The listing builds one solid part. Answer for the finished solid, in the listing's coordinates (mm). A direction names the side the tool comes from. Give positions to 0.01 mm unless a question says otherwise; leave off trailing zeros. Loops run counter-clockwise (first coordinate to the right, second up) from the corner with the lowest first, then second, coordinate; pieces in that order, holes last. Notation, with made-up numbers: M -39.5,22.25 L -5.5,22.25 A28 cw -5.5,44.25 Z; hole C 13.25,59 d6. An arc over 180 degrees is marked long. Use one line per item in the form item = value. Start each with the question number.
1. The part is cut by section C-C (y = -4.5). Write down the section's boundary in (x, z), and give its area (3 significant figures).
2. The part is cut by section D-D (z = -25.5). Write down the section's boundary in (x, y), and give its area (3 significant figures).
3. The part is cut by section A-A (x = -39). Write down the section's boundary in (y, z), and give its area (3 significant figures).
4. Each of these flat-tipped pins is pushed along its axis until it touches: pin 1 Ø3 at (y, z) = (-6.5, -50) entering from +X; pin 2 Ø6 at (y, z) = (-6.5, -80.5) entering from +X; pin 3 Ø19.5 at (x, z) = (39, -25.5) entering from +Y; pin 4 Ø6 at (y, z) = (-7, -113.5) entering from -X. Where does it stop, or does it pass through?
5. The part is cut by section B-B (z = -117.5). Write down the section's boundary in (x, y).
6. For faces 1 (the face through (29, -6, -129.5)), 2 (the face through (68.797, -6.084, -1.141)), 3 (the face through (-17, -6, -105.5)), 4 (the face through (50.5, -6, -89)), 5 (the face through (-50.5, -6, -89)), determine the directions among +Z, -Z, +X, -X, +Y, -Y from which every point of the face is accessible in a straight line to the end or side of a thin tool.
7. Straight lines are drawn through the part: line 1 (Z direction, x = -15.5, y = -8.75); line 2 (X direction, y = -1.5, z = -25); line 3 (Z direction, x = 26.5, y = -4.5). For each, find the intervals that lie inside material, in ascending order. Write a range as from..to.
8. The mould has two halves that part along Z. Classify faces 6 (the face through (-11.5, -6, -118)), 7 (the face through (51.703, -6.084, -51.141)), 8 (the face through (0, -6, -84.6)), 9 (the face through (27.216, -5.916, -112.047)): released by +Z, released by -Z, zero draft, split by the parting line, or undercut.
from build123d import *

# Parameters (mm, degrees)
F0_R     = 5.5
F0_R_2   = 7.55
F1_DEPTH = 12
F2_R     = 4


with BuildPart() as f1:
    # F0 (on Front) → F1 (new body)
    with BuildSketch(Plane.XZ):
        Polygon((0, -84.6), (0, 0), (-70, 0), (-70, -50), (-50.5, -50), (-50.5, -129.5), (-11.5, -129.5), (-11.5, -105.5), (-22.5, -105.5), (-22.5, -84.6), align=None)
        with Locations((-26.5, -117.5)):
            Circle(F0_R, mode=Mode.SUBTRACT)
        with Locations((-39, -25.5)):
            Circle(F0_R_2, mode=Mode.SUBTRACT)
    extrude(amount=F1_DEPTH)

    # F2
    f2_edges = [f1.edges().sort_by_distance(p)[0] for p in [
        (-50.5, -6, -129.5),
        (-50.5, -6, -50),
        (-70, -6, -50),
        (-70, -6, 0),
    ]]
    fillet(f2_edges, radius=F2_R)

    # F3: F1 across face


with BuildPart() as f1_1:
    add(f1.part)
    add(f1.part.mirror(Plane(origin=(0, -6, -42.3), x_dir=(0, 1, 0), z_dir=(1, 0, 0))))


solid = f1_1.part
Derived:
q1.outline = M -70,-46 A4 ccw -66,-50 L -54.5,-50 A4 cw -50.5,-54 L -50.5,-125.5 A4 ccw -46.5,-129.5 L -11.5,-129.5 L -11.5,-105.5 L -22.5,-105.5 L -22.5,-84.6 L 22.5,-84.6 L 22.5,-105.5 L 11.5,-105.5 L 11.5,-129.5 L 46.5,-129.5 A4 ccw 50.5,-125.5 L 50.5,-54 A4 cw 54.5,-50 L 66,-50 A4 ccw 70,-46 L 70,-4 A4 ccw 66,0 L -66,0 A4 ccw -70,-4 Z; hole C -39,-25.5 d15.1; hole C -26.5,-117.5 d11; hole C 26.5,-117.5 d11; hole C 39,-25.5 d15.1
q1.area = 13,000 mm2
q2.outline = M -70,-12 L -46.55,-12 L -46.55,0 L -70,0 Z; M -31.45,-12 L 31.45,-12 L 31.45,0 L -31.45,0 Z; M 46.55,-12 L 70,-12 L 70,0 L 46.55,0 Z
q2.area = 1,320 mm2
q3.outline = M -12,-129.5 L 0,-129.5 L 0,-33.05 L -12,-33.05 Z; M -12,-17.95 L 0,-17.95 L 0,0 L -12,0 Z
q3.area = 1,370 mm2
q4.pin_1 = 69.12
q4.pin_2 = 50.5
q4.pin_3 = 0
q4.pin_4 = -50.5
q5.outline = M -50.5,-12 L -32,-12 L -32,0 L -50.5,0 Z; M -21,-12 L -11.5,-12 L -11.5,0 L -21,0 Z; M 11.5,-12 L 21,-12 L 21,0 L 11.5,0 Z; M 32,-12 L 50.5,-12 L 50.5,0 L 32,0 Z
q6.face_1 = -Z, +X, -X, +Y, -Y
q6.face_2 = +Z, +X, +Y, -Y
q6.face_3 = +Y, -Y
q6.face_4 = -Z, +X, +Y, -Y
q6.face_5 = -Z, -X, +Y, -Y
q7.line_1 = -129.5..-105.5, -84.6..0
q7.line_2 = -70..-46.53, -31.47..31.47, 46.53..70
q7.line_3 = -129.5..-123, -112..0
q8.face_6 = zero draft
q8.face_7 = released by -Z
q8.face_8 = undercut
q8.face_9 = undercut
